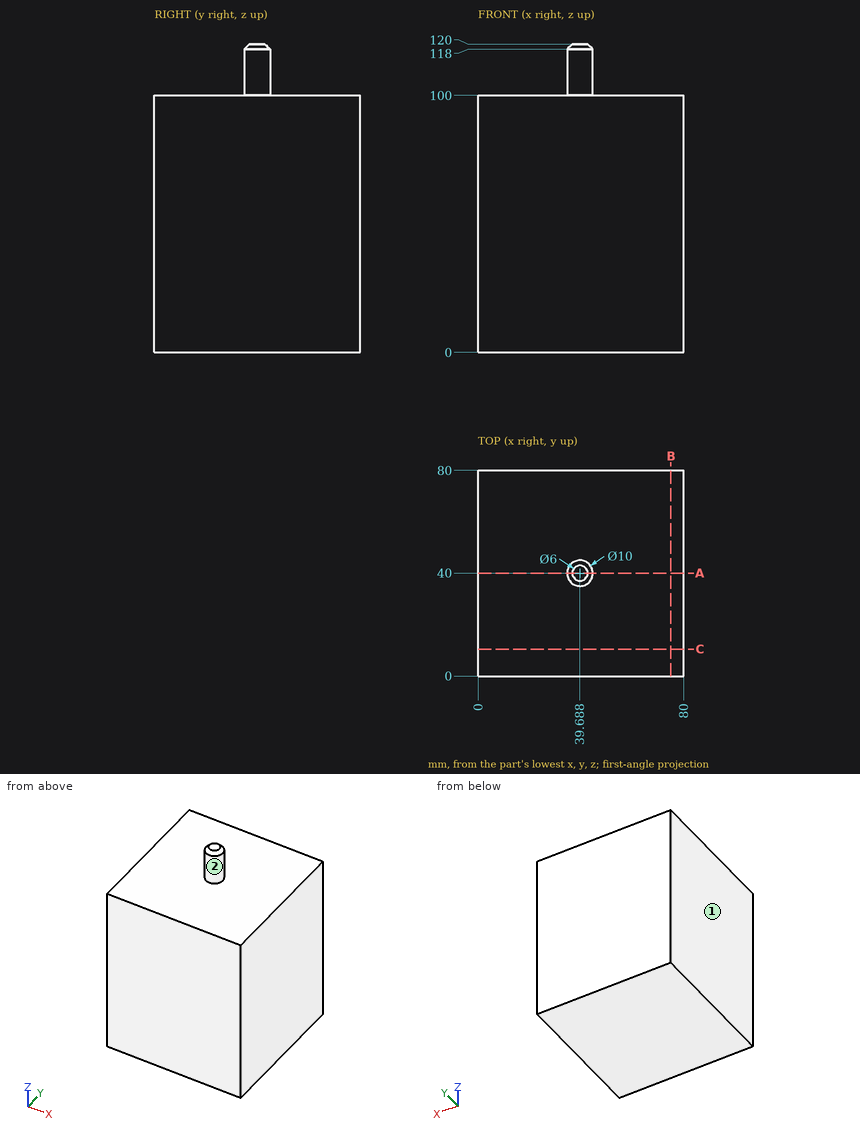
For this review, use the dimensioned drawing (mm, ordinates from the lowest corner) and the shaded views. A direction names the side the tool comes from. Round coordinates to 2 decimals unless told otherwise and drop trailing zeros. Write each loop counter-clockwise with the first axis right and the second up, starting at its lowest first coordinate (ties: lowest second). Pieces come first, ordered by that corner, then holes. Notation, with made-up numbers: (-1, 50) - (6, 50) arc R19 ccw to (6, 83) - close; hole circle Ø6 at (-28, 72.5). An arc over 180 degrees is marked (long way). Use a Markdown table: item, result.
Q1. We need section A-A (y = 40). Give the boundary of the cut face in (x, z), plus the area to 3 significant figures.
Derived:
| item | result |
|---|---|
| outline | (0, 0) - (80, 0) - (80, 100) - (44.69, 100) - (44.69, 118) - (42.69, 120) - (36.69, 120) - (34.69, 118) - (34.69, 100) - (0, 100) - close |
| area | 8,200 mm2 |
Q2. Wall thickness on line 1 along Z through (x, y) = (26.5, 28): over which ranges is the line inside the solid? List them lowest first.
Derived:
| item | result |
|---|---|
| line 1 | z = 0 to 100 |
Q3. We need section B-B (x = 75). Give the boundary of the cut face in (y, z).
Derived:
| item | result |
|---|---|
| outline | (0, 0) - (80, 0) - (80, 100) - (0, 100) - close |
Q4. Machinability: for the marked faces 1 and 2, which of the approach directions +Z, -Z, +X, -X, +Y, -Y give a long, thin tool a straight path to every point of the face, cutting with its end or side? Answer none if there is none.
Derived:
| item | result |
|---|---|
| face 1 | +Z, -Z, -X, +Y, -Y |
| face 2 | +Z |
